Can you work these out from the model? Positions are in its coordinate system, mm. A direction names the side the tool comes from. Give positions to 0.01 mm unless a question says otherwise; leave off trailing zeros. Write each loop counter-clockwise with the first axis right and the second up, starting at its lowest first coordinate (ties: lowest second). Pieces come first, ordered by that corner, then holes.
```python
from build123d import *

# Parameters (mm, degrees)
SKETCH1_W           = 304.8
SKETCH1_H           = 76.2
BOSS_EXTRUDE1_DEPTH = 1
SKETCH2_W           = 304.8
SKETCH2_H           = 1
EXTRUDE_THIN1_DEPTH = 20
SKETCH5_W           = 304.8
SKETCH5_H           = 1
EXTRUDE_THIN2_DEPTH = 20


with BuildPart() as part:
    # Sketch1 → Boss-Extrude1 (new body)
    with BuildSketch(Plane(origin=(0, 0, 0), x_dir=(1, 0, 0), z_dir=(0, 1, 0))):
        Rectangle(SKETCH1_W, SKETCH1_H)
    extrude(amount=BOSS_EXTRUDE1_DEPTH)

    # Sketch2 → Extrude-Thin1 (add)
    with BuildSketch(Plane(origin=(0, 1, 0), x_dir=(1, 0, 0), z_dir=(0, 1, 0))):
        with Locations((0, -37.6)):
            Rectangle(SKETCH2_W, SKETCH2_H)
    extrude(amount=EXTRUDE_THIN1_DEPTH)

    # Sketch5 → Extrude-Thin2 (add)
    with BuildSketch(Plane(origin=(0, 1, 0), x_dir=(1, 0, 0), z_dir=(0, 1, 0))):
        with Locations((0, 37.6)):
            Rectangle(SKETCH5_W, SKETCH5_H)
    extrude(amount=EXTRUDE_THIN2_DEPTH)


solid = part.part
```
1) For pin 1 Ø8 at (x, z) = (28.5, -28.5) entering from +Y; pin 2 Ø12 at (x, z) = (-113.5, 19) entering from -Y; pin 3 Ø2 at (y, z) = (3, 12) entering from -X, each with a flat end and sliding along its axis, tell me the tip position at first contact or that it passes through.
Values follow:
pin 1: stops at y = 1
pin 2: stops at y = 0
pin 3: passes through
2) Please list where these lines run through material, in increasing order: L1, parallel to Z at x = -101, y = 16.5; L2, parallel to Y at x = 91.5, z = 25.5.
Values follow:
L1: z = -38.1 to -37.1, 37.1 to 38.1
L2: y = 0 to 1
3) If we mould it in two halves opening along Z, with no side actions, what happens to faces 3 (the face through (-2, 0, -1)), 4 (the face through (-2, 10, 38.1)), 5 (the face through (-2, 11, -37.1)), 6 (the face through (-2, 10, -38.1))? For each: +Z half, -Z half, draft (parallel to the pull), parting line (faces both ways), or undercut.
Values follow:
face 3: draft
face 4: +Z half
face 5: undercut
face 6: -Z half
4) Suppose I cut it at A-A on y = 12.5. Write out the boundary of the cut face in (x, z).
Values follow:
outline: (-152.4, -38.1) - (152.4, -38.1) - (152.4, -37.1) - (-152.4, -37.1) - close; (-152.4, 37.1) - (152.4, 37.1) - (152.4, 38.1) - (-152.4, 38.1) - close
5) For faces 1 (the face through (-152.4, 0.3, 0.2)), 2 (the face through (-2, 11, 37.1)), which set-ups out of +Z, -Z, +X, -X, +Y, -Y let a thin tool reach every point of the face, with its end or its side?
Values follow:
face 1: +Z, -Z, -X, +Y, -Y
face 2: +X, -X, +Y
6) Suppose I cut it at B-B on x = 132. Write out the boundary of the cut face in (y, z).
Values follow:
outline: (0, -38.1) - (21, -38.1) - (21, -37.1) - (1, -37.1) - (1, 37.1) - (21, 37.1) - (21, 38.1) - (0, 38.1) - close
7) Suppose I cut it at C-C on z = 13.5. Write out the boundary of the cut face in (x, y), plus the area to 3 significant figures.
Values follow:
outline: (-152.4, 0) - (152.4, 0) - (152.4, 1) - (-152.4, 1) - close
area: 305 mm2
